```python
from build123d import *

# Parameters (mm, degrees)
SKETCH1_W           = 96
SKETCH1_H           = 2
BOSS_EXTRUDE1_DEPTH = 98
SKETCH2_W           = 10
SKETCH2_H           = 2
BOSS_EXTRUDE2_DEPTH = 2
SKETCH3_W           = 10
SKETCH3_H           = 2
BOSS_EXTRUDE3_DEPTH = 2
SKETCH4_W           = 10
SKETCH4_H           = 2
BOSS_EXTRUDE4_DEPTH = 2
FILLET1_R           = 0.5


with BuildPart() as part:
    # Sketch1 → Boss-Extrude1 (new body)
    with BuildSketch(Plane.XY):
        with Locations((0, 49)):
            Rectangle(SKETCH1_W, SKETCH1_H)
    extrude(amount=BOSS_EXTRUDE1_DEPTH)

    # Sketch2 → Boss-Extrude2 (add)
    with BuildSketch(Plane(origin=(0, 0, 0), x_dir=(-1, 0, 0), z_dir=(0, 0, -1))):
        with Locations((-23, 49)):
            Rectangle(SKETCH2_W, SKETCH2_H)
    boss_extrude2 = extrude(amount=BOSS_EXTRUDE2_DEPTH)

    # Mirror1: Boss-Extrude2 across plane
    add(boss_extrude2.mirror(Plane(origin=(0, 0, 0), x_dir=(0, 0, 1), z_dir=(1, 0, 0))))

    # Sketch3 → Boss-Extrude3 (add)
    with BuildSketch(Plane.ZY.offset(48)):
        with Locations((73, 49)):
            Rectangle(SKETCH3_W, SKETCH3_H)
    boss_extrude3 = extrude(amount=BOSS_EXTRUDE3_DEPTH)

    # Mirror2: Boss-Extrude3 across plane
    add(boss_extrude3.mirror(Plane.XY.offset(50)))

    # Sketch4 → Boss-Extrude4 (add)
    with BuildSketch(Plane(origin=(48, 0, 0), x_dir=(0, 0, -1), z_dir=(1, 0, 0))):
        with Locations((-73, 49)):
            Rectangle(SKETCH4_W, SKETCH4_H)
    boss_extrude4 = extrude(amount=BOSS_EXTRUDE4_DEPTH)

    # Mirror3: Boss-Extrude4 across plane
    add(boss_extrude4.mirror(Plane.XY.offset(50)))

    # Fillet1
    fillet1_edges = [part.edges().sort_by_distance(p)[0] for p in [
        (18, 49, -2),
        (28, 49, -2),
        (-28, 49, -2),
        (-18, 49, -2),
        (-50, 49, 68),
        (-50, 49, 78),
        (-50, 49, 22),
        (-50, 49, 32),
        (50, 49, 78),
        (50, 49, 68),
        (50, 49, 32),
        (50, 49, 22),
    ]]
    fillet(fillet1_edges, radius=FILLET1_R)


solid = part.part
```
The listing builds one solid part. Answer for the finished solid, in the listing's coordinates (mm). Coordinates: 2 decimals unless noted, no trailing zeros. Order: outer loops, then holes, each group sorted by start corner. A loop starts at its lowest first (then second) coordinate and runs counter-clockwise, first axis right, second up. Notation, with made-up numbers: M 42.25,-24.75 L 99.25,-24.75 A23 cw 99.25,-8.75 Z; hole C 10.25,-19.5 d5. An arc over 180 degrees is marked long. Answer as a JSON object with one key per item and string values. Group by question number.
1. Straight lines are drawn through the part: line 1 (Z direction, x = -9, y = 49.6); line 2 (X direction, y = 48.45, z = 80.5). For each, find the intervals that lie inside material, in ascending order.
2. Section A-A on z = 10 is taken. Write down the section's boundary in (x, y).
3. Flat-ended cylindrical pins translate along their axes: P1, Ø0.8, axis at x = 48.5, y = 48.5, coming from the +Z side; P2, Ø0.6, axis at x = 2, y = 49, coming from the -Z side; P3, Ø1, axis at y = 49.5, z = 11.5, coming from the +X side. Find the tip coordinate at first contact, or state that the pin passes through.
4. Section B-B on x = -6 is taken. Write down the section's boundary in (y, z), then the cut area to 3 significant figures.
Values follow:
{
 "1": {"line 1": "0 to 98", "line 2": "-48 to 48"},
 "2": {"outline": "M -48,48 L 48,48 L 48,50 L -48,50 Z"},
 "3": {"P1": "z = 78", "P2": "z = 0", "P3": "x = 48"},
 "4": {"outline": "M 48,0 L 50,0 L 50,98 L 48,98 Z", "area": "196 mm2"}
}
